Geometry check sheet. Reference: the model listing, model coordinates, mm. Coordinates: 2 decimals unless noted, no trailing zeros. Loops run counter-clockwise (first coordinate to the right, second up) from the corner with the lowest first, then second, coordinate; pieces in that order, holes last.
Autodesk Inventor part; units mm, degrees
ref_plane "YZ Plane" through (0, 0, 0) normal (1, 0, 0) x (0, 1, 0)
ref_plane "XZ Plane" through (0, 0, 0) normal (0, 1, 0) x (-1, 0, 0)
ref_plane "XY Plane" through (0, 0, 0) normal (0, 0, 1) x (1, 0, 0)
sketch "Sketch1" plane through (0, 0, 0) normal (1, 0, 0) x (0, 1, 0)
  line L0 (0, 8.6387) -> (0, -8.0216)
  line L1 (-27.4792, 0) -> (24.1471, 0)
  circle A0 centre (-46.5, 0) radius 2.7
  circle A1 centre (46.5, 0) radius 2.7
  arc A2 (42.0088, -6.2545) -> (42.0088, 6.2545) centre (46.5, 0) ccw
  arc A3 (-42.0088, 6.2545) -> (-42.0088, -6.2545) centre (-46.5, 0) ccw
  line L2 (0, 2.5) -> (30.3433, 2.5)
  line L3 (0, 2.5) -> (-30.3433, 2.5)
  line L4 (0, -2.5) -> (-30.3433, -2.5)
  line L5 (0, -2.5) -> (30.3433, -2.5)
  arc A4 (30.3433, 2.5) -> (42.0088, 6.2545) centre (30.3433, 22.5) ccw
  arc A5 (42.0088, -6.2545) -> (30.3433, -2.5) centre (30.3433, -22.5) ccw
  arc A6 (-42.0088, 6.2545) -> (-30.3433, 2.5) centre (-30.3433, 22.5) ccw
  arc A7 (-30.3433, -2.5) -> (-42.0088, -6.2545) centre (-30.3433, -22.5) ccw
  point P0 (0, 0)
  point P1 (46.5, -7.7)
  point P2 (46.5, 7.7)
  point P3 (-46.5, -7.7)
  point P4 (-46.5, 7.7)
  point P5 (-39.2171, 2.5)
  point P6 (-39.2171, -2.5)
  point P7 (39.2171, -2.5)
  point P8 (39.2171, 2.5)
  dimension "d5" = 93
  dimension "d3" = 5
  dimension "d2" = 5
  dimension "d4" = 5.4
  dimension "d1" = 5
  dimension "d0" = 20
extrude "Extrusion1" add sketch "Sketch1" along normal blind 3
fillet "Fillet1" radius 1 4 edges at (3, 43.8, 0) (0, 43.8, 0) (3, -49.2, 0) (0, -49.2, 0)
properties part number "ön differansiyel"
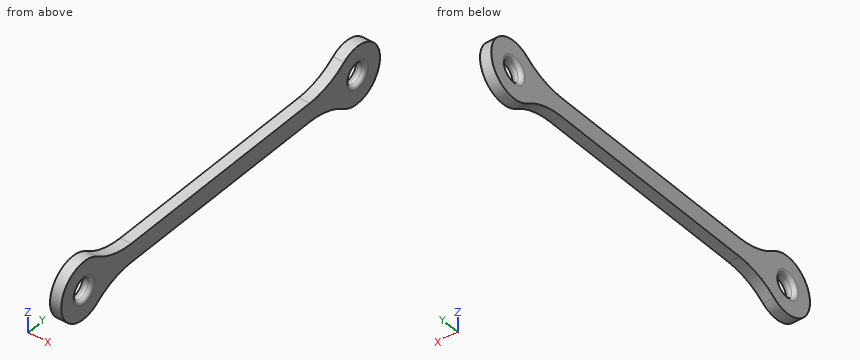
(1) Sectioned sample at C-C on y = -7. Record the cut outline in (x, z).
Findings:
outline: (0, -2.5) - (3, -2.5) - (3, 2.5) - (0, 2.5) - close
(2) Sectioned sample at A-A on y = 46.5. Record the cut outline in (x, z), and give its area (3 significant figures).
Findings:
outline: (0, -7.7) - (3, -7.7) - (3, -3.7) arc R1 ccw to (2, -2.7) - (1, -2.7) arc R1 ccw to (0, -3.7) - close; (0, 3.7) arc R1 ccw to (1, 2.7) - (2, 2.7) arc R1 ccw to (3, 3.7) - (3, 7.7) - (0, 7.7) - close
area: 29.1 mm2
(3) Scan lines: L1, parallel to Z at x = 1.45, y = -46.5; L2, parallel to Y at x = 1.05, z = 2; L3, parallel to Y at x = 2, z = 1.5 (3 decimals). Record each from-to range of solid material in increasing order.
Findings:
L1: z = -7.7 to -2.7, 2.7 to 7.7
L2: y = -53.94 to -48.31, -44.69 to 44.69, 48.31 to 53.94
L3: y = -54.052 to -48.745, -44.255 to 44.255, 48.745 to 54.052
(4) Gauge pin test, flat ends, axial feed: pin 1 Ø3 at (y, z) = (-46.5, 0) entering from -X; pin 2 Ø1.5 at (x, y) = (2, 6.5) entering from +Z. Record the tip position at first contact, or that the pin passes through.
Findings:
pin 1: passes through
pin 2: stops at z = 2.5
(5) Sectioned sample at D-D on y = 34.5. Record the cut outline in (x, z).
Findings:
outline: (0, -2.94) - (3, -2.94) - (3, 2.94) - (0, 2.94) - close
(6) Sectioned sample at B-B on z = 0. Record the cut outline in (x, y).
Findings:
outline: (0, -54.2) - (3, -54.2) - (3, -50.2) arc R1 ccw to (2, -49.2) - (1, -49.2) arc R1 ccw to (0, -50.2) - close; (0, -42.8) arc R1 ccw to (1, -43.8) - (2, -43.8) arc R1 ccw to (3, -42.8) - (3, 42.8) arc R1 ccw to (2, 43.8) - (1, 43.8) arc R1 ccw to (0, 42.8) - close; (0, 50.2) arc R1 ccw to (1, 49.2) - (2, 49.2) arc R1 ccw to (3, 50.2) - (3, 54.2) - (0, 54.2) - close
